Here's how the part is built. I have some questions about the finished solid (model axes, mm). Face numbers are marked on the shaded views. Round coordinates to 2 decimals unless told otherwise and drop trailing zeros. Write each loop counter-clockwise with the first axis right and the second up, starting at its lowest first coordinate (ties: lowest second). Pieces come first, ordered by that corner, then holes. Notation, with made-up numbers: (-25, -30.75) -> (25, -30.75) arc R15 ccw to (25, -19.75) -> close; hole circle Ø6 at (1, 48). An arc over 180 degrees is marked (long way). Answer as CSV lines item,"result".
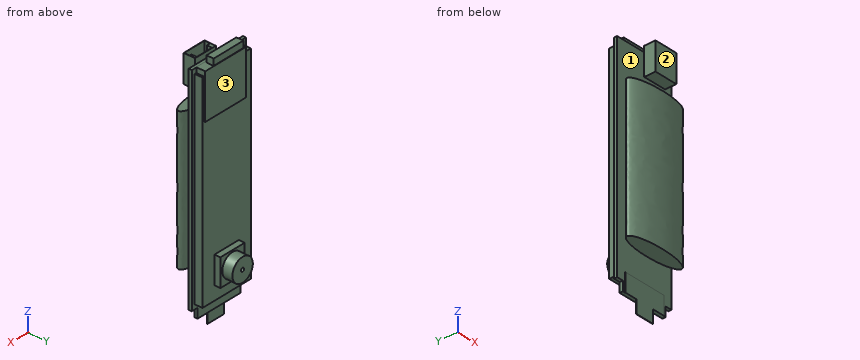
```python
from build123d import *

# Parameters (mm, degrees)
BOSS_EXTRUDE2_DEPTH      = 6.35
BOSS_EXTRUDE2_DEPTH_BACK = 6.35
BOSS_EXTRUDE2_START      = 15.24
SKETCH4_W                = 12.7
SKETCH4_H                = 1.397
BOSS_EXTRUDE3_DEPTH      = 22.86
BOSS_EXTRUDE3_DEPTH_BACK = 22.86
SKETCH5_RX               = 10.033
SKETCH5_RY               = 2.589631332
BOSS_EXTRUDE4_DEPTH      = 36.4109
BOSS_EXTRUDE4_DEPTH_BACK = 36.4109
SKETCH6_W                = 19.9136
SKETCH6_H                = 1.016
SKETCH7_W                = 14.992697908
SKETCH7_H                = 14.648957972
BOSS_EXTRUDE6_DEPTH      = 2.921
SKETCH10_W               = 10.922
SKETCH10_H               = 2.286
BOSS_EXTRUDE7_DEPTH      = 2.115042028
CUT_EXTRUDE1_REACH       = 42.496
SKETCH11_W               = 2.0828
SKETCH11_H               = 3.1369
SKETCH12_W               = 7.62
SKETCH12_H               = 9.017
BOSS_EXTRUDE8_DEPTH      = 3.683
SKETCH13_W               = 8.89
SKETCH13_H               = 8.89
BOSS_EXTRUDE9_DEPTH      = 4.445
SKETCH14_R               = 3.748513876
BOSS_EXTRUDE10_DEPTH     = 3.302
SKETCH15_R               = 0.573513876
CUT_EXTRUDE2_DEPTH       = 3.302
SKETCH16_W               = 14.224
SKETCH16_H               = 5.9309
SKETCH16_W_2             = 6.096
SKETCH16_H_2             = 4.2291
BOSS_EXTRUDE11_DEPTH     = 0.127
CUT_EXTRUDE3_DEPTH       = 6.35
SKETCH18_W               = 8.89
SKETCH18_H               = 8.89
BOSS_EXTRUDE13_DEPTH     = 2.54


with BuildPart() as part:
    # Sketch4 → Boss-Extrude2 (new, two sides: drawn at the far end of the back side and taken through both)
    with BuildSketch(Plane.XY.offset(BOSS_EXTRUDE2_START - BOSS_EXTRUDE2_DEPTH_BACK)):
        with Locations((0, -1.2065)):
            Rectangle(SKETCH4_W, SKETCH4_H)
    extrude(amount=BOSS_EXTRUDE2_DEPTH + BOSS_EXTRUDE2_DEPTH_BACK)

    # Sketch5 → Boss-Extrude3 (add, two sides: drawn at the far end of the back side and taken through both)
    with BuildSketch(Plane.XY.offset(-BOSS_EXTRUDE3_DEPTH_BACK)):
        with Locations((0, -3.81)):
            Ellipse(SKETCH5_RX, SKETCH5_RY)
    extrude(amount=BOSS_EXTRUDE3_DEPTH + BOSS_EXTRUDE3_DEPTH_BACK)

    # Sketch6 → Boss-Extrude4 (add, two sides: drawn at the far end of the back side and taken through both)
    with BuildSketch(Plane.XY.offset(-BOSS_EXTRUDE4_DEPTH_BACK)):
        Rectangle(SKETCH6_W, SKETCH6_H)
    extrude(amount=BOSS_EXTRUDE4_DEPTH + BOSS_EXTRUDE4_DEPTH_BACK)

    # Sketch7 → Boss-Extrude6 (add)
    with BuildSketch(Plane(origin=(0, 0.508, 0), x_dir=(1, 0, 0), z_dir=(0, 1, 0))):
        with Locations((0.809451046, -29.181178986)):
            Rectangle(SKETCH7_W, SKETCH7_H)
    extrude(amount=BOSS_EXTRUDE6_DEPTH)

    # Sketch10 → Boss-Extrude7 (add)
    with BuildSketch(Plane.XY.offset(36.505657972)):
        with Locations((-0.381, 2.159)):
            Rectangle(SKETCH10_W, SKETCH10_H)
    extrude(amount=BOSS_EXTRUDE7_DEPTH)

    # Sketch11 → Cut-Extrude1 (cut, up to next)
    with BuildSketch(Plane(origin=(0, 0.508, 0), x_dir=(1, 0, 0), z_dir=(0, 1, 0)), mode=Mode.PRIVATE) as cut_extrude1_sk1:
        with Locations((-8.9154, 34.84245)):
            Rectangle(SKETCH11_W, SKETCH11_H)
    cut_extrude1_tool1 = extrude(cut_extrude1_sk1.sketch, amount=-CUT_EXTRUDE1_REACH, mode=Mode.PRIVATE) & part.part
    # Sketch11 → Cut-Extrude1 (cut, up to next)
    with BuildSketch(Plane(origin=(0, 0.508, 0), x_dir=(1, 0, 0), z_dir=(0, 1, 0)), mode=Mode.PRIVATE) as cut_extrude1_sk2:
        with Locations((8.9154, 34.84245)):
            Rectangle(SKETCH11_W, SKETCH11_H)
    cut_extrude1_tool2 = extrude(cut_extrude1_sk2.sketch, amount=-CUT_EXTRUDE1_REACH, mode=Mode.PRIVATE) & part.part
    add(cut_extrude1_tool1.solids().sort_by_distance((-8.9154, 0.508, -34.84245))[0], mode=Mode.SUBTRACT)
    add(cut_extrude1_tool2.solids().sort_by_distance((8.9154, 0.508, -34.84245))[0], mode=Mode.SUBTRACT)

    # Sketch12 → Boss-Extrude8 (add)
    with BuildSketch(Plane.XZ.offset(0.508)):
        with Locations((3.81, 33.8074)):
            Rectangle(SKETCH12_W, SKETCH12_H)
    extrude(amount=BOSS_EXTRUDE8_DEPTH)

    # Sketch13 → Boss-Extrude9 (add)
    with BuildSketch(Plane(origin=(0, 0.508, 0), x_dir=(1, 0, 0), z_dir=(0, 1, 0))):
        with Locations((0, 22.86)):
            Rectangle(SKETCH13_W, SKETCH13_H)
    extrude(amount=BOSS_EXTRUDE9_DEPTH)

    # Sketch14 → Boss-Extrude10 (add)
    with BuildSketch(Plane(origin=(0, 4.953, 0), x_dir=(1, 0, 0), z_dir=(0, 1, 0))):
        with Locations(Location((0, 22.733, 0), (0, 0, 90))):
            Circle(SKETCH14_R)
    extrude(amount=BOSS_EXTRUDE10_DEPTH)

    # Sketch15 → Cut-Extrude2 (cut)
    with BuildSketch(Plane(origin=(0, 8.255, 0), x_dir=(1, 0, 0), z_dir=(0, 1, 0))):
        with Locations(Location((0, 22.733, 0), (0, 0, 270))):
            Circle(SKETCH15_R)
    extrude(amount=-CUT_EXTRUDE2_DEPTH, mode=Mode.SUBTRACT)

    # Sketch16 → Boss-Extrude11 (add)
    with BuildSketch(Plane.XZ.offset(0.508)):
        with Locations((0, -33.44545)):
            Rectangle(SKETCH16_W, SKETCH16_H)
        with Locations((0, -38.52545)):
            Rectangle(SKETCH16_W_2, SKETCH16_H_2)
    extrude(amount=BOSS_EXTRUDE11_DEPTH)

    # Sketch17 → Cut-Extrude3 (cut)
    with BuildSketch(Plane.XY.offset(38.3159)):
        Polygon((1.305274753, -0.6096), (6.889189319, -0.6096), (6.889189319, -2.287768833), (7.5438, -2.287768833), (7.5438, -4.1148), (0.0762, -4.1148), (0.0762, -2.287768833), (1.305274753, -2.287768833), align=None)
    extrude(amount=-CUT_EXTRUDE3_DEPTH, mode=Mode.SUBTRACT)

    # Sketch18 → Boss-Extrude13 (add)
    with BuildSketch(Plane(origin=(0, 0.508, 0), x_dir=(1, 0, 0), z_dir=(0, 1, 0))):
        Polygon((8.3058, -34.838229956), (8.89, -34.838229956), (8.89, 31.75), (-8.89, 31.75), (-8.89, -34.838229956), (-6.686897908, -34.838229956), (-6.686897908, -21.8567), (8.3058, -21.8567), align=None)
        with Locations((0, 22.86)):
            Rectangle(SKETCH18_W, SKETCH18_H, mode=Mode.SUBTRACT)
    extrude(amount=BOSS_EXTRUDE13_DEPTH)


solid = part.part
```
1. Suppose I cut it at A-A on z = -24.5. Please give me the cut outline in (x, y) (3 decimals), and give its area (3 significant figures).
Numbers:
outline,"(-9.957, -0.508) -> (9.957, -0.508) -> (9.957, 0.508) -> (8.89, 0.508) -> (8.89, 3.048) -> (4.445, 3.048) -> (4.445, 4.953) -> (3.306, 4.953) -> (3.306, 8.255) -> (-3.306, 8.255) -> (-3.306, 4.953) -> (-4.445, 4.953) -> (-4.445, 3.048) -> (-8.89, 3.048) -> (-8.89, 0.508) -> (-9.957, 0.508) -> close"
area,"104 mm^2"
2. If I drill on line 1 (Z direction, x = 1.5, y = -2.5); line 2 (X direction, y = 7.25, z = -22.5); line 3 (X direction, y = 0, z = 20), over which ranges is the centre line in solid material (lowest first)?
Numbers:
line 1,"z = -22.86 to 22.86, 29.3 to 31.97"
line 2,"x = -3.74 to -0.52, 0.52 to 3.74"
line 3,"x = -9.96 to 9.96"
3. For pin 1 Ø0.8 at (x, y) = (9, 0) entering from -Z; pin 2 Ø0.9 at (y, z) = (-3, 35) entering from -X; pin 3 Ø1.1 at (x, z) = (-2.5, 37) entering from -Y, each with a flat end and sliding along its axis, tell me the tip position at first contact or that it passes through.
Numbers:
pin 1,"stops at z = -33.27"
pin 2,"stops at x = 0"
pin 3,"stops at y = 0.51"
4. If we mould it in two halves opening along Y, with no side actions, what happens to the marked faces 1, 2 and 3? For each: released by +Y, released by -Y, zero draft, split by the parting line, or undercut.
Numbers:
face 1,"undercut"
face 2,"released by -Y"
face 3,"released by +Y"
